Answer from the drawing. Dimensions are ordinates in mm from the lowest x, y and z of the part. Round coordinates to 2 decimals unless told otherwise and drop trailing zeros. Order: outer loops, then holes, each group sorted by start corner. A loop starts at its lowest first (then second) coordinate and runs counter-clockwise, first axis right, second up. Notation, with made-up numbers: (46, -14) - (56, -14) arc R17 cw to (56, 14) - close; hole circle Ø3 at (27.5, -15). An arc over 180 degrees is marked (long way). One line per question, with ' | ' between items. Start each with the question number.
1) The part is cut by section A-A, the plane x = 3.5. Give the vertices of the cut face in (y, z) (1 decimal).
2) Straight lines are drawn through the part: line 1 (Z direction, x = 5.75, y = 7.5); line 2 (Y direction, x = 2.5, z = 8.25); line 3 (Z direction, x = 3.25, y = 6). For each, find the intervals that lie inside material, in ascending order. Write a range as from..to.
3) Flat-ended cylindrical pins translate along their axes: pin 1 (2 mm diameter, centred on x = 6, z = 3.5, fed in from +Y); pin 2 (5.5 mm diameter, centred on y = 7.51, z = 6.5, fed in from +X). Find the tip coordinate at first contact, or state that the pin passes through.
4) The mould has two halves that part along Z. Classify the marked faces 1, 2, 3 and 4: pulls with the +Z half, pulls with the -Z half, needs draft (parallel to the pull), parting line crosses it, or undercut.
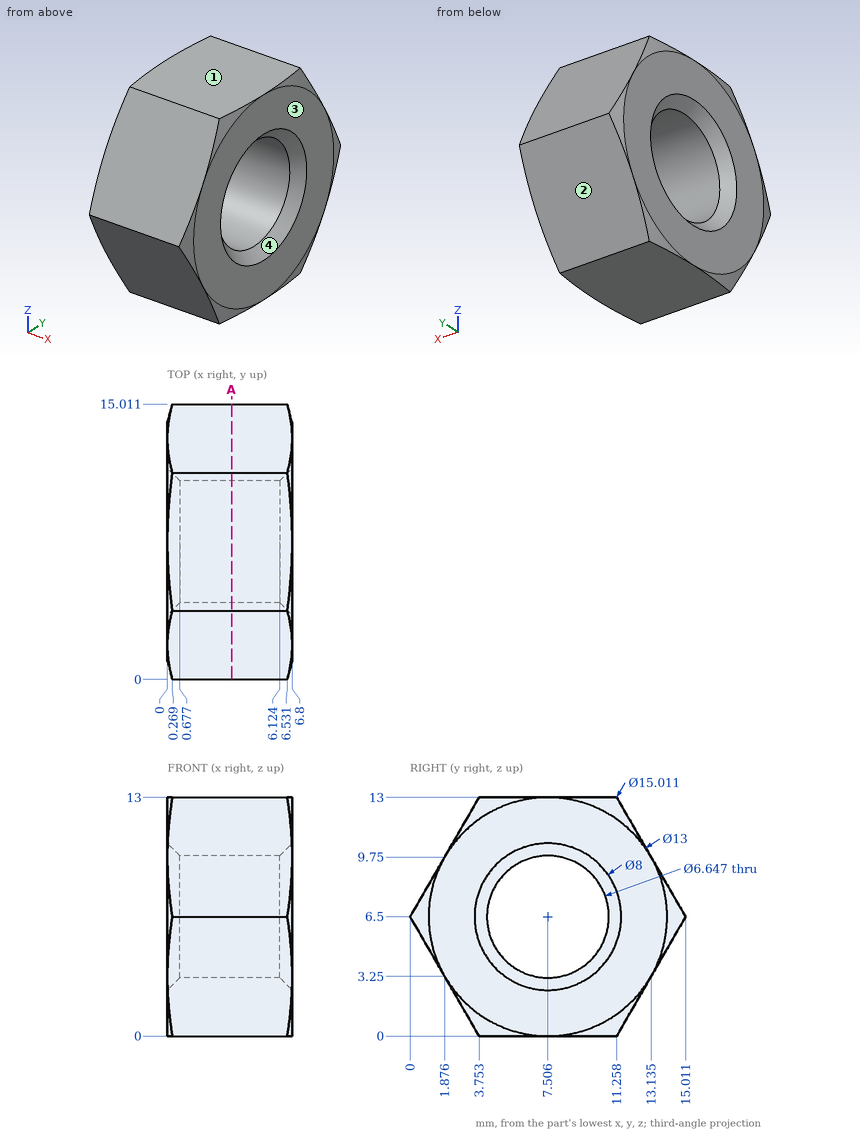
Values:
1) outline: (0, 6.5) - (3.8, 0) - (11.3, 0) - (15, 6.5) - (11.3, 13) - (3.8, 13) - close; hole circle Ø6.6 at (7.5, 6.5)
2) line 1: z = 0..3.18, 9.82..13 | line 2: y = 1.01..4.68, 10.33..14 | line 3: z = 0..3.54, 9.46..13
3) pin 1: stops at y = 13.86 | pin 2: passes through
4) face 1: pulls with the +Z half | face 2: pulls with the -Z half | face 3: needs draft | face 4: undercut
